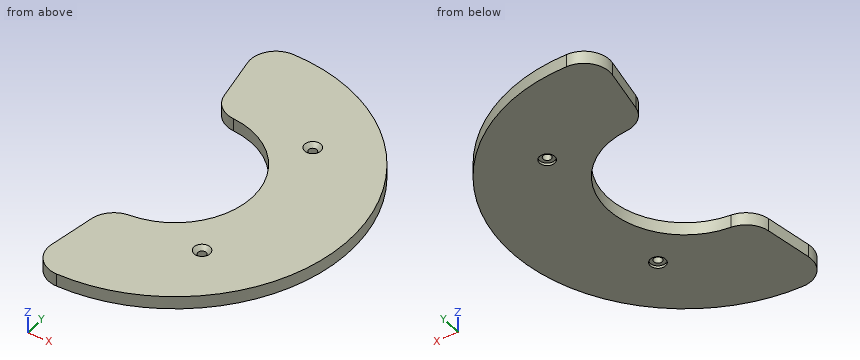
from build123d import *

# Parameters (mm, degrees)
SKETCH_1_R                   = 1.6
EXTRUDE_1_DEPTH              = 5
FILLET_1_R                   = 10
HOLE_WIZARD_M3_1_D           = 3.2
HOLE_WIZARD_M3_1_CSINK_D     = 6.3
HOLE_WIZARD_M3_1_CSINK_ANGLE = 90
SKETCH_5_R                   = 3
CUT_EXTRUDE_1_DEPTH          = 1


with BuildPart() as part:
    # ｽｹｯﾁ1 → ﾎﾞｽ - 押し出し1 (new body)
    with BuildSketch(Plane.XY):
        with BuildLine():
            Line((-5.20944533, 29.54423259), (-11.808076081, 66.966927205))
            ThreePointArc((-11.808076081, 66.966927205), (68, 0), (-11.808076081, -66.966927205))
            Line((-11.808076081, -66.966927205), (-5.20944533, -29.54423259))
            ThreePointArc((-5.20944533, -29.54423259), (30, 0), (-5.20944533, 29.54423259))
        make_face()
        with Locations((31.819805153, 31.819805153)):
            Circle(SKETCH_1_R, mode=Mode.SUBTRACT)
        with Locations(Location((31.819805153, -31.819805153, 0), (0, 0, 180))):
            Circle(SKETCH_1_R, mode=Mode.SUBTRACT)
    extrude(amount=EXTRUDE_1_DEPTH)

    # ﾌｨﾚｯﾄ1
    fillet_1_edges = [part.edges().sort_by_distance(p)[0] for p in [
        (-11.808076081, -66.966927205, 2.5),
        (-5.20944533, -29.54423259, 2.5),
        (-5.20944533, 29.54423259, 2.5),
        (-11.808076081, 66.966927205, 2.5),
    ]]
    fillet(fillet_1_edges, radius=FILLET_1_R)

    # M3 丸皿ねじ用皿穴1 (through all)
    with Locations(Plane.XY.offset(5)):
        with Locations((31.819805153, 31.819805153), (31.819805153, -31.819805153)):
            CounterSinkHole(HOLE_WIZARD_M3_1_D / 2, HOLE_WIZARD_M3_1_CSINK_D / 2, counter_sink_angle=HOLE_WIZARD_M3_1_CSINK_ANGLE)

    # ｽｹｯﾁ5 → ｶｯﾄ - 押し出し1 (cut)
    with BuildSketch(Plane(origin=(0, 0, 0), x_dir=(-1, 0, 0), z_dir=(0, 0, -1))):
        with Locations((-31.819805153, 31.819805153)):
            Circle(SKETCH_5_R)
        with Locations(Location((-31.819805153, -31.819805153, 0), (0, 0, 180))):
            Circle(SKETCH_5_R)
    extrude(amount=-CUT_EXTRUDE_1_DEPTH, mode=Mode.SUBTRACT)


solid = part.part
Can you work these out from the model? Positions are in its coordinate system, mm. Give positions to 0.01 mm unless a question says otherwise; leave off trailing zeros. Order: outer loops, then holes, each group sorted by start corner. A loop starts at its lowest first (then second) coordinate and runs counter-clockwise, first axis right, second up. Notation, with made-up numbers: M -2.5,7.25 L 5.5,7.25 A13 cw 5.5,15.25 Z; hole C 44,19 d5. An arc over 180 degrees is marked long. Use a Markdown table: item, result. Add a question column.
Item 1: Will these pins go through, and if not, where does the flat tip stop? pin 1 (2 mm diameter, centred on x = 43, z = 1.5, fed in from -Y); pin 2 (5 mm diameter, centred on x = 31.82, y = -31.82, fed in from +Z); pin 3 (3 mm diameter, centred on y = 34, z = 2.5, fed in from -X).
Item 2: If I drill on L1, parallel to Y at x = 26.5, z = 0.9; L2, parallel to Y at x = 18.5, z = 0.65; L3, parallel to X at y = -1, z = 0.45, over which ranges is the centre line in solid material (lowest first)? Write a range as [from, to].
Item 3: Suppose I cut it at A-A (x = -2.5). List the corners of the cut face in (y, z) for me.
Item 4: Suppose I cut it at D-D (x = 15). List the corners of the cut face in (y, z) for me.
Item 5: Suppose I cut it at C-C (y = 0). List the corners of the cut face in (x, z) for me, then the cut area to 3 significant figures.
Item 6: Suppose I cut it at B-B (z = 2.05). List the corners of the cut face in (x, y) for me, then the cut area to 3 significant figures.
Answer sheet:
| question | item | result |
|---|---|---|
| 1 | pin 1 | stops at y = -53.48 |
| 1 | pin 2 | stops at z = 4.35 |
| 1 | pin 3 | stops at x = -5.87 |
| 2 | L1 | y = [-62.62, -14.06], [14.06, 62.62] |
| 2 | L2 | y = [-65.44, -23.62], [23.62, 65.44] |
| 2 | L3 | x = [29.98, 67.99] |
| 3 | outline | M -67.7,0 L -31.61,0 L -31.61,5 L -67.7,5 Z; M 31.61,0 L 67.7,0 L 67.7,5 L 31.61,5 Z |
| 4 | outline | M -66.32,0 L -25.98,0 L -25.98,5 L -66.32,5 Z; M 25.98,0 L 66.32,0 L 66.32,5 L 25.98,5 Z |
| 5 | outline | M 30,0 L 68,0 L 68,5 L 30,5 Z |
| 5 | area | 190 mm² |
| 6 | outline | M -9.92,-56.26 A10 ccw -0.09,-68 A68 ccw -0.09,68 A10 ccw -9.92,56.26 L -6.73,38.14 A10 ccw 2.34,29.91 A30 cw 2.34,-29.91 A10 ccw -6.73,-38.14 Z; hole C 31.82,-31.82 d3.2; hole C 31.82,31.82 d3.2 |
| 6 | area | 6,400 mm² |
